Can you work these out from the model? Positions are in its coordinate system, mm. Face numbers are marked on the shaded views. Coordinates: 2 decimals unless noted, no trailing zeros. Order: outer loops, then holes, each group sorted by start corner. A loop starts at its lowest first (then second) coordinate and runs counter-clockwise, first axis right, second up. Notation, with made-up numbers: (14, -33) - (60, -33) arc R21 ccw to (60, -10) - close; hole circle Ø7 at (4.5, 46). An arc over 180 degrees is marked (long way). Use a Markdown table: item, result. Add a question column.
(1) I want a section at B-B (z = 0). List the corners of the cut face in (x, y) for me, and give its area (3 significant figures).
(2) We'd pull the mould along Z, two halves only. Please class the marked faces 1, 2, 3 and 4: pulls with the +Z half, pulls with the -Z half, needs draft (parallel to the pull), parting line crosses it, or undercut.
(3) If I drill on L1, parallel to Z at x = 0, y = -0.35; L2, parallel to X at y = -0.05, z = 0; L3, parallel to X at y = 0.1, z = 1, over which ranges is the centre line in solid material (lowest first)? Write a range as [from, to].
(4) I want a section at D-D (x = -4). List the corners of the cut face in (y, z) for me.
(5) I want a section at A-A (x = 0). List the corners of the cut face in (y, z) for me, and give its area (3 significant figures).
(6) I want a section at C-C (y = -0.95). List the corners of the cut face in (x, z) for me, and give its area (3 significant figures).
```python
from build123d import *

# Parameters (mm, degrees)
SKETCH1_R           = 2.0828
BOSS_EXTRUDE1_DEPTH = 1.5875
FILLET1_R           = 1
CHAMFER1_SIZE       = 0.2


with BuildPart() as part:
    # Sketch1 → Boss-Extrude1 (new body, symmetric)
    with BuildSketch(Plane(origin=(0, 0, 0), x_dir=(1, 0, 0), z_dir=(0, 1, 0))):
        Polygon((2.520494769, 4.365625), (-2.520494769, 4.365625), (-5.040989538, 0), (-2.520494769, -4.365625), (2.520494769, -4.365625), (5.040989538, 0), align=None)
        Circle(SKETCH1_R, mode=Mode.SUBTRACT)
    extrude(amount=BOSS_EXTRUDE1_DEPTH, both=True)

    # Fillet1
    fillet1_edges = [part.edges().sort_by_distance(p)[0] for p in [
        (5.040989538, 0, 0),
        (2.520494769, 0, 4.365625),
        (-2.520494769, 0, 4.365625),
        (-5.040989538, 0, 0),
        (-2.520494769, 0, -4.365625),
        (2.520494769, 0, -4.365625),
    ]]
    fillet(fillet1_edges, radius=FILLET1_R)

    # Chamfer1
    chamfer1_edges = [part.edges().sort_by_distance(p)[0] for p in [
        (-2.0828, -1.5875, 0),
        (-2.0828, 1.5875, 0),
        (3.780742153, -1.5875, -2.1828125),
        (3.780742153, 1.5875, -2.1828125),
        (3.780742153, -1.5875, 2.1828125),
        (0, -1.5875, 4.365625),
        (-3.780742153, -1.5875, 2.1828125),
        (-3.780742153, -1.5875, -2.1828125),
        (0, -1.5875, -4.365625),
        (-2.4431445, -1.5875, 4.231650404),
        (2.4431445, -1.5875, -4.231650404),
        (-2.4431445, -1.5875, -4.231650404),
        (-4.886288999, -1.5875, 0),
        (2.4431445, -1.5875, 4.231650404),
        (4.886288999, -1.5875, 0),
        (3.780742153, 1.5875, 2.1828125),
        (0, 1.5875, -4.365625),
        (-3.780742153, 1.5875, -2.1828125),
        (-3.780742153, 1.5875, 2.1828125),
        (0, 1.5875, 4.365625),
        (-2.4431445, 1.5875, 4.231650404),
        (2.4431445, 1.5875, -4.231650404),
        (-2.4431445, 1.5875, -4.231650404),
        (-4.886288999, 1.5875, 0),
        (2.4431445, 1.5875, 4.231650404),
        (4.886288999, 1.5875, 0),
    ]]
    chamfer(chamfer1_edges, length=CHAMFER1_SIZE)


solid = part.part
```
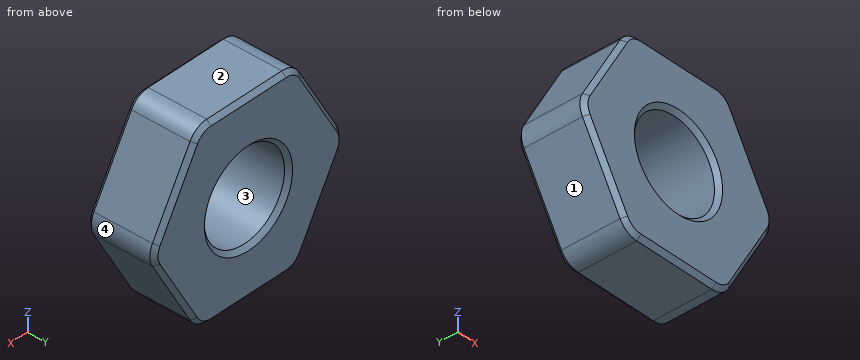
Answers follow:
| question | item | result |
|---|---|---|
| 1 | outline | (-4.89, -1.39) - (-4.69, -1.59) - (-2.28, -1.59) - (-2.08, -1.39) - (-2.08, 1.39) - (-2.28, 1.59) - (-4.69, 1.59) - (-4.89, 1.39) - close; (2.08, -1.39) - (2.28, -1.59) - (4.69, -1.59) - (4.89, -1.39) - (4.89, 1.39) - (4.69, 1.59) - (2.28, 1.59) - (2.08, 1.39) - close |
| 1 | area | 17.6 mm² |
| 2 | face 1 | pulls with the -Z half |
| 2 | face 2 | pulls with the +Z half |
| 2 | face 3 | undercut |
| 2 | face 4 | parting line crosses it |
| 3 | L1 | z = [-4.37, -2.08], [2.08, 4.37] |
| 3 | L2 | x = [-4.89, -2.08], [2.08, 4.89] |
| 3 | L3 | x = [-4.46, -1.83], [1.83, 4.46] |
| 4 | outline | (-1.59, -1.4) - (-1.39, -1.8) - (1.39, -1.8) - (1.59, -1.4) - (1.59, 1.4) - (1.39, 1.8) - (-1.39, 1.8) - (-1.59, 1.4) - close |
| 5 | outline | (-1.59, -4.17) - (-1.39, -4.37) - (1.39, -4.37) - (1.59, -4.17) - (1.59, -2.28) - (1.39, -2.08) - (-1.39, -2.08) - (-1.59, -2.28) - close; (-1.59, 2.28) - (-1.39, 2.08) - (1.39, 2.08) - (1.59, 2.28) - (1.59, 4.17) - (1.39, 4.37) - (-1.39, 4.37) - (-1.59, 4.17) - close |
| 5 | area | 14.3 mm² |
| 6 | outline | (-4.75, -0.5) - (-2.81, -3.87) arc R1 ccw to (-1.94, -4.37) - (1.94, -4.37) arc R1 ccw to (2.81, -3.87) - (4.75, -0.5) arc R1 ccw to (4.75, 0.5) - (2.81, 3.87) arc R1 ccw to (1.94, 4.37) - (-1.94, 4.37) arc R1 ccw to (-2.81, 3.87) - (-4.75, 0.5) arc R1 ccw to start; hole circle Ø4.17 at (0, 0) |
| 6 | area | 52.1 mm² |
